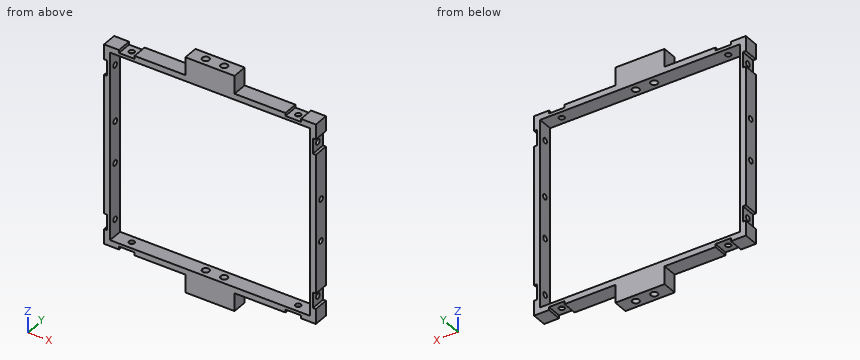
```python
from build123d import *

# Parameters (mm, degrees)
SKETCH1_W           = 71
SKETCH1_H           = 67
SKETCH1_W_2         = 67
SKETCH1_H_2         = 63
BOSS_EXTRUDE1_DEPTH = 5
SKETCH2_R           = 0.9
CUT_EXTRUDE1_DEPTH  = 121
SKETCH3_R           = 1
CUT_EXTRUDE2_DEPTH  = 0.01
SKETCH9_W           = 5.2
SKETCH9_H           = 5
CUT_EXTRUDE6_DEPTH  = 1
SKETCH10_W          = 5.2
SKETCH10_H          = 5
CUT_EXTRUDE7_DEPTH  = 1
SKETCH11_R          = 0.9
CUT_EXTRUDE8_DEPTH  = 81
SKETCH12_R          = 0.9
CUT_EXTRUDE9_DEPTH  = 81
SKETCH14_R          = 1.15
CUT_EXTRUDE10_DEPTH = 79
SKETCH15_W          = 16.483338106
SKETCH15_H          = 5
BOSS_EXTRUDE2_DEPTH = 6
SKETCH16_R          = 1.15
CUT_EXTRUDE11_DEPTH = 30
SKETCH17_R          = 1.15
CUT_EXTRUDE12_DEPTH = 30


with BuildPart() as part:
    # Sketch1 → Boss-Extrude1 (new body)
    with BuildSketch(Plane(origin=(0, 0, 0), x_dir=(1, 0, 0), z_dir=(0, 1, 0))):
        Rectangle(SKETCH1_W, SKETCH1_H)
        Rectangle(SKETCH1_W_2, SKETCH1_H_2, mode=Mode.SUBTRACT)
    extrude(amount=BOSS_EXTRUDE1_DEPTH)

    # Sketch2 → Cut-Extrude1 (cut)
    with BuildSketch(Plane(origin=(35.5, 0, 0), x_dir=(0, 0, -1), z_dir=(1, 0, 0))):
        with Locations((-6.999701476, 2.591425228)):
            Circle(SKETCH2_R)
        with Locations((7, 2.5)):
            Circle(SKETCH2_R)
    extrude(amount=-CUT_EXTRUDE1_DEPTH, mode=Mode.SUBTRACT)

    # Sketch3 → Cut-Extrude2 (cut)
    with BuildSketch(Plane.XY.offset(33.5)):
        with Locations((0, 2.5)):
            Circle(SKETCH3_R)
    extrude(amount=-CUT_EXTRUDE2_DEPTH, mode=Mode.SUBTRACT)

    # Sketch9 → Cut-Extrude6 (cut)
    with BuildSketch(Plane.XY.offset(33.5)):
        with Locations((-27.9, 2.5)):
            Rectangle(SKETCH9_W, SKETCH9_H)
        with Locations((27.9, 2.5)):
            Rectangle(SKETCH9_W, SKETCH9_H)
    cut_extrude6 = extrude(amount=-CUT_EXTRUDE6_DEPTH, mode=Mode.SUBTRACT)

    # Sketch10 → Cut-Extrude7 (cut)
    with BuildSketch(Plane(origin=(35.5, 0, 0), x_dir=(0, 0, -1), z_dir=(1, 0, 0))):
        with Locations((-25.9, 2.5)):
            Rectangle(SKETCH10_W, SKETCH10_H)
        with Locations((25.9, 2.5)):
            Rectangle(SKETCH10_W, SKETCH10_H)
    cut_extrude7 = extrude(amount=-CUT_EXTRUDE7_DEPTH, mode=Mode.SUBTRACT)

    # Mirror2: Cut-Extrude7 across plane
    add(cut_extrude7.mirror(Plane(origin=(0, 0, 0), x_dir=(0, 0, 1), z_dir=(1, 0, 0))), mode=Mode.SUBTRACT)

    # Mirror3: Cut-Extrude6 across plane
    add(cut_extrude6.mirror(Plane.XY), mode=Mode.SUBTRACT)

    # Sketch11 → Cut-Extrude8 (cut)
    with BuildSketch(Plane(origin=(34.5, 0, 0), x_dir=(0, 0, -1), z_dir=(1, 0, 0))):
        with Locations((25.9, 2.5)):
            Circle(SKETCH11_R)
        with Locations((-25.9, 2.5)):
            Circle(SKETCH11_R)
    extrude(amount=-CUT_EXTRUDE8_DEPTH, mode=Mode.SUBTRACT)

    # Sketch12 → Cut-Extrude9 (cut)
    with BuildSketch(Plane.XY.offset(32.5)):
        with Locations((27.9, 2.5)):
            Circle(SKETCH12_R)
        with Locations((-27.9, 2.5)):
            Circle(SKETCH12_R)
    extrude(amount=-CUT_EXTRUDE9_DEPTH, mode=Mode.SUBTRACT)

    # Sketch14 → Cut-Extrude10 (cut)
    with BuildSketch(Plane(origin=(0, 0, -33.5), x_dir=(-1, 0, 0), z_dir=(0, 0, -1))):
        with Locations((-3.085, 2.5)):
            Circle(SKETCH14_R)
        with Locations((3.088228318, 2.5)):
            Circle(SKETCH14_R)
    cut_extrude10 = extrude(amount=-CUT_EXTRUDE10_DEPTH, mode=Mode.SUBTRACT)

    # Sketch15 → Boss-Extrude2 (add)
    with BuildSketch(Plane(origin=(0, 0, -33.5), x_dir=(-1, 0, 0), z_dir=(0, 0, -1))):
        with Locations((0, 2.5)):
            Rectangle(SKETCH15_W, SKETCH15_H)
    boss_extrude2 = extrude(amount=BOSS_EXTRUDE2_DEPTH)

    # Sketch16 → Cut-Extrude11 (cut)
    with BuildSketch(Plane.XY.offset(-31.5)):
        with Locations((-3.088228318, 2.5)):
            Circle(SKETCH16_R)
        with Locations((3.085, 2.5)):
            Circle(SKETCH16_R)
    extrude(amount=-CUT_EXTRUDE11_DEPTH, mode=Mode.SUBTRACT)

    # Mirror4: Cut-Extrude10, Boss-Extrude2 across plane
    add(cut_extrude10.mirror(Plane.XY), mode=Mode.SUBTRACT)
    add(boss_extrude2.mirror(Plane.XY))

    # Sketch17 → Cut-Extrude12 (cut)
    with BuildSketch(Plane(origin=(0, 0, 31.5), x_dir=(-1, 0, 0), z_dir=(0, 0, -1))):
        with Locations((-3.085, 2.5)):
            Circle(SKETCH17_R)
        with Locations((3.088228318, 2.5)):
            Circle(SKETCH17_R)
    extrude(amount=-CUT_EXTRUDE12_DEPTH, mode=Mode.SUBTRACT)


solid = part.part
```
The model under review builds one solid part; all positions refer to its coordinate system, in mm. Round coordinates to 2 decimals unless told otherwise and drop trailing zeros. Loops run counter-clockwise (first coordinate to the right, second up) from the corner with the lowest first, then second, coordinate; pieces in that order, holes last. Notation, with made-up numbers: (-8.75, 3.5) - (-4.75, 3.5) arc R11 ccw to (-4.75, 24.5) - close; hole circle Ø8 at (65.5, -17.5). An arc over 180 degrees is marked (long way). Use a Markdown table: item, result. Add a question column.
Q1. Add section B-B (x = -27.9). State the section outline as (y, z) points, plus the area to 3 significant figures.
Q2. Add section A-A (x = 0). State how many separate pieces and enclosed holes the cut face has, plus the area to 3 significant figures.
Q3. Add section C-C (z = -13.5). State the section outline as (x, y) points, plus the area to 3 significant figures.
Q4. Insertion check: pin 1 Ø3 at (x, y) = (-17, 2.5) entering from -Z; pin 2 Ø1.1 at (x, y) = (-35, 3.5) entering from +Z; pin 3 Ø1.5 at (y, z) = (1.5, -27) entering from -X. Each pin has a flat end and moves straight along its axis. Give the tip position at first contact, or say it passes through.
Q5. For probe 1 along X at (y, z) = (1.55, -6.5); probe 2 along Z at (x, y) = (-11.5, 4.3); probe 3 along Z at (x, y) = (5, 3.6), list the stretches that pass through material, from the lowest coordinate up.
Q6. Add section D-D (x = 17). State the section outline as (y, z) points.
Worked answers:
| question | item | result |
|---|---|---|
| 1 | outline | (0, -32.5) - (1.6, -32.5) - (1.6, -31.5) - (0, -31.5) - close; (0, 31.5) - (1.6, 31.5) - (1.6, 32.5) - (0, 32.5) - close; (3.4, -32.5) - (5, -32.5) - (5, -31.5) - (3.4, -31.5) - close; (3.4, 31.5) - (5, 31.5) - (5, 32.5) - (3.4, 32.5) - close |
| 1 | area | 6.40 mm² |
| 2 | separate pieces | 2 |
| 2 | enclosed holes | 1 |
| 2 | area | 80.0 mm² |
| 3 | outline | (-35.5, 0) - (-33.5, 0) - (-33.5, 5) - (-35.5, 5) - close; (33.5, 0) - (35.5, 0) - (35.5, 5) - (33.5, 5) - close |
| 3 | area | 20.0 mm² |
| 4 | pin 1 | z = -33.5 |
| 4 | pin 2 | z = 33.5 |
| 4 | pin 3 | x = -34.5 |
| 5 | probe 1 | -35.5 to -33.5, 33.5 to 35.5 |
| 5 | probe 2 | -33.5 to -31.5, 31.5 to 33.5 |
| 5 | probe 3 | -39.5 to -31.5, 31.5 to 39.5 |
| 6 | outline | (0, -33.5) - (5, -33.5) - (5, -31.5) - (0, -31.5) - close; (0, 31.5) - (5, 31.5) - (5, 33.5) - (0, 33.5) - close |
